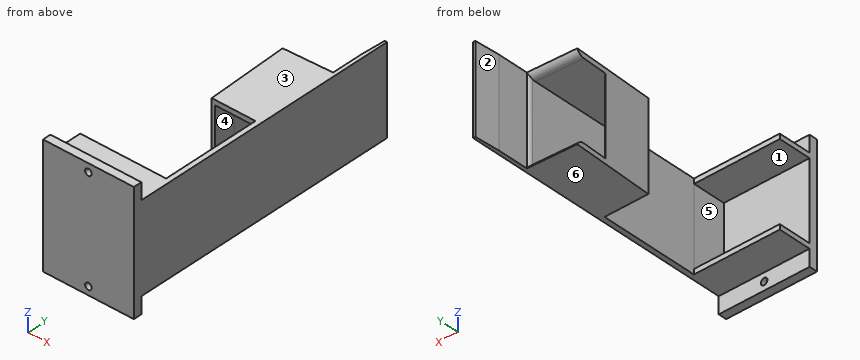
```python
from build123d import *

# Parameters (mm, degrees)
CROQUIS1_W              = 55
CROQUIS1_H              = 53
CROQUIS1_W_2            = 48.773584906
CROQUIS1_H_2            = 47
SALIENTE_EXTRUIR1_DEPTH = 25
SALIENTE_EXTRUIR2_DEPTH = 160
SALIENTE_EXTRUIR3_DEPTH = 50
SALIENTE_EXTRUIR5_DEPTH = 3
CROQUIS4_W              = 100
CROQUIS4_H              = 30
CORTAR_EXTRUIR1_DEPTH   = 63
CHAFL_N1_SIZE           = 2
CHAFL_N1_SIZE2          = 57.272506566
CROQUIS1_2_W            = 55
CROQUIS1_2_H            = 53
CROQUIS1_2_W_2          = 48.773584906
CROQUIS1_2_H_2          = 47
SALIENTE_EXTRUIR6_DEPTH = 5
CROQUIS5_W              = 30
CROQUIS5_H              = 60
CORTAR_EXTRUIR2_DEPTH   = 60
CROQUIS1_4_W            = 55
CROQUIS1_4_H            = 10
CROQUIS1_4_R            = 2
SALIENTE_EXTRUIR7_DEPTH = 5
CROQUIS6_W              = 53
CROQUIS6_H              = 15
CORTAR_EXTRUIR3_DEPTH   = 5
CHAFL_N2_SIZE           = 30
CHAFL_N2_SIZE_2         = 1.572233378
CHAFL_N3_SIZE           = 5
CHAFL_N3_SIZE2          = 0.881634904
CROQUIS7_W              = 47
CROQUIS7_H              = 20
CORTAR_EXTRUIR4_DEPTH   = 40
CROQUIS8_W              = 47
CROQUIS8_H              = 40
CORTAR_EXTRUIR5_DEPTH   = 10
CORTAR_EXTRUIR6_DEPTH   = 70
REDONDEO3_R             = 5
REDONDEO5_R             = 5


with BuildPart() as part:
    # Croquis1 → Saliente-Extruir1 (new body)
    with BuildSketch(Plane(origin=(0, 0, 0), x_dir=(1, 0, 0), z_dir=(0, 1, 0))):
        Rectangle(CROQUIS1_W, CROQUIS1_H)
        Rectangle(CROQUIS1_W_2, CROQUIS1_H_2, mode=Mode.SUBTRACT)
    extrude(amount=SALIENTE_EXTRUIR1_DEPTH)

    # Croquis2 → Saliente-Extruir2 (add)
    with BuildSketch(Plane(origin=(0, 25, 0), x_dir=(1, 0, 0), z_dir=(0, 1, 0))):
        Polygon((0, 23.5), (0, 26.5), (27.5, 26.5), (27.5, -26.5), (0, -26.5), (0, -23.5), (24.386792453, -23.5), (24.386792453, 23.5), align=None)
    extrude(amount=SALIENTE_EXTRUIR2_DEPTH)



with BuildPart() as body_2:
    # Croquis3 → Saliente-Extruir3 (new body)
    with BuildSketch(Plane(origin=(0, 0, 23.5), x_dir=(-1, 0, 0), z_dir=(0, 0, -1))):
        Polygon((0, 155), (5, 155), (2, 85), (0, 85), align=None)
    extrude(amount=SALIENTE_EXTRUIR3_DEPTH)


with BuildPart() as part_1:
    add(part.part)

    add(body_2.part)  # Saliente-Extruir5 merges body 2
    # Croquis3<4> → Saliente-Extruir5 (add)
    with BuildSketch(Plane(origin=(0, 0, 23.5), x_dir=(-1, 0, 0), z_dir=(0, 0, -1))):
        Polygon((0, 155), (5, 155), (2, 85), (0, 85), align=None)
    extrude(amount=-SALIENTE_EXTRUIR5_DEPTH)

    # Croquis4 → Cortar-Extruir1 (cut)
    with BuildSketch(Plane(origin=(0, 0, -26.5), x_dir=(-1, 0, 0), z_dir=(0, 0, -1))):
        with Locations((25.5, 170)):
            Rectangle(CROQUIS4_W, CROQUIS4_H)
    extrude(amount=-CORTAR_EXTRUIR1_DEPTH, mode=Mode.SUBTRACT)

    # Chaflán1
    chafl_n1_edges = [part_1.edges().sort_by_distance(p)[0] for p in [
        (0, 155, 0),
    ]]
    chafl_n1_side = [part_1.faces().sort_by_distance(p)[0] for p in [
        (9.75, 155, -25.893431785),
    ]]
    chamfer(chafl_n1_edges, length=CHAFL_N1_SIZE, length2=CHAFL_N1_SIZE2, reference=chafl_n1_side[0])

    # Croquis1<2> → Saliente-Extruir6 (add)
    # profile 1 of 2: a face of its own
    with BuildSketch(Plane(origin=(0, 0, 0), x_dir=(1, 0, 0), z_dir=(0, 1, 0))):
        Rectangle(CROQUIS1_2_W, CROQUIS1_2_H)
        Rectangle(CROQUIS1_2_W_2, CROQUIS1_2_H_2, mode=Mode.SUBTRACT)
    # profile 2 of 2: a face of its own
    with BuildSketch(Plane(origin=(0, 0, 0), x_dir=(1, 0, 0), z_dir=(0, 1, 0))):
        Rectangle(CROQUIS1_2_W_2, CROQUIS1_2_H_2)
    extrude(amount=SALIENTE_EXTRUIR6_DEPTH)

    # Croquis5 → Cortar-Extruir2 (cut)
    with BuildSketch(Plane(origin=(0, 0, -26.5), x_dir=(-1, 0, 0), z_dir=(0, 0, -1))):
        with Locations((-9.5, 55)):
            Rectangle(CROQUIS5_W, CROQUIS5_H)
    extrude(amount=-CORTAR_EXTRUIR2_DEPTH, mode=Mode.SUBTRACT)

    # Croquis1<4> → Saliente-Extruir7 (add)
    # profile 1 of 2: a face of its own
    with BuildSketch(Plane(origin=(0, 0, 0), x_dir=(1, 0, 0), z_dir=(0, 1, 0))):
        with Locations((0, 31.5)):
            Rectangle(CROQUIS1_4_W, CROQUIS1_4_H)
        with Locations(Location((0, 31.5, 0), (0, 0, 270))):
            Circle(CROQUIS1_4_R, mode=Mode.SUBTRACT)
    # profile 2 of 2: a face of its own
    with BuildSketch(Plane(origin=(0, 0, 0), x_dir=(1, 0, 0), z_dir=(0, 1, 0))):
        with Locations((0, -31.5)):
            Rectangle(CROQUIS1_4_W, CROQUIS1_4_H)
        with Locations(Location((0, -31.5, 0), (0, 0, 270))):
            Circle(CROQUIS1_4_R, mode=Mode.SUBTRACT)
    extrude(amount=SALIENTE_EXTRUIR7_DEPTH)

    # Croquis6 → Cortar-Extruir3 (cut)
    with BuildSketch(Plane.ZY.offset(-24.5)):
        with Locations((0, 177.5)):
            Rectangle(CROQUIS6_W, CROQUIS6_H)
    extrude(amount=-CORTAR_EXTRUIR3_DEPTH, mode=Mode.SUBTRACT)

    # Chaflán2
    # the kernel refuses this chamfer: 30, 1.572233378 mm, written as the material it takes off along each edge
    with BuildSketch(Plane(origin=(24.5, 170, -104.496046635), x_dir=(-0.002013023422382327, -0.9999979738662979, 0), z_dir=(0, 0, 1))) as chafl_n2_piece_1_section:
        Polygon((CHAFL_N2_SIZE * 0.999997973866, CHAFL_N2_SIZE * 0.00201302342238), (-CHAFL_N2_SIZE_2 * 0.00201302342301, CHAFL_N2_SIZE_2 * 0.999997974179), (0, 0), align=None)
    chafl_n2_piece_1 = extrude(amount=208.992093269, mode=Mode.PRIVATE)
    chafl_n2_piece_1 = split(chafl_n2_piece_1, bisect_by=Plane(origin=(25.111424092, 155, 0), z_dir=(0, 1, 0)), keep=Keep.TOP, mode=Mode.PRIVATE)
    add(chafl_n2_piece_1, mode=Mode.SUBTRACT)

    # Chaflán3
    chafl_n3_edges = [part_1.edges().sort_by_distance(p)[0] for p in [
        (24.386792453, 155, 0),
    ]]
    chafl_n3_side = [part_1.faces().sort_by_distance(p)[0] for p in [
        (24.386792453, 120, 0),
    ]]
    chamfer(chafl_n3_edges, length=CHAFL_N3_SIZE, length2=CHAFL_N3_SIZE2, reference=chafl_n3_side[0])

    # Croquis7 → Cortar-Extruir4 (cut)
    with BuildSketch(Plane.ZY.offset(27.5)):
        with Locations((0, 15)):
            Rectangle(CROQUIS7_W, CROQUIS7_H)
    extrude(amount=-CORTAR_EXTRUIR4_DEPTH, mode=Mode.SUBTRACT)

    # Croquis8 → Cortar-Extruir5 (cut)
    with BuildSketch(Plane(origin=(1.639845182, 0.070279079, 0), x_dir=(0, 0, 1), z_dir=(-0.9990828958176697, -0.04281783839218585, 0))):
        with Locations((0, 135.071938044)):
            Rectangle(CROQUIS8_W, CROQUIS8_H)
    extrude(amount=-CORTAR_EXTRUIR5_DEPTH, mode=Mode.SUBTRACT)

    # Croquis9 → Cortar-Extruir6 (cut)
    with BuildSketch(Plane.XY.offset(26.5)):
        Polygon((-5, 155), (25.286116689, 155), (25.286116689, 136.279617509), (-4.143643232, 135.018342084), align=None)
    extrude(amount=-CORTAR_EXTRUIR6_DEPTH, mode=Mode.SUBTRACT)

    # Redondeo3
    # the kernel refuses this fillet: 5 mm, written as the material it takes off along each edge
    with BuildSketch(Plane(origin=(-4.143643232, 135.018342084, 23.5), x_dir=(0, 0, 1), z_dir=(0.9990828958176697, 0.042817838392185704, 0))) as redondeo3_piece_1_section:
        with BuildLine():
            CenterArc((5, 4.582575695), REDONDEO3_R, 180, 66.421821522)
            Line((0, 4.582575695), (-0.1, 4.582575695))
            Line((-0.1, 4.582575695), (-0.1, 0))
            Line((-0.1, 0), (0, -0.1))
            ThreePointArc((0, -0.1), (1.5, -0.1), (2.96, -0.091651514))
            Line((2.96, -0.091651514), (3, 0))
        make_face()
    redondeo3_piece_1 = extrude(amount=40.013064323, mode=Mode.PRIVATE)
    redondeo3_piece_1 = split(redondeo3_piece_1, bisect_by=Plane(origin=(24.386792453, 134.515316135, 24.276456874), z_dir=(-1, 0, 0)), keep=Keep.TOP, mode=Mode.PRIVATE)
    add(redondeo3_piece_1, mode=Mode.SUBTRACT)
    with BuildSketch(Plane(origin=(24.386792453, 136.241075042, 23.5), x_dir=(0.9990828958176863, 0.04281783839180005, 0), z_dir=(0, 0, -1))) as redondeo3_piece_2:
        with BuildLine():
            CenterArc((4.874569404, 3.033807599), REDONDEO3_R, 182.454031675, 34.901674654)
            Line((-0.120845075, 2.819718407), (-0.220753364, 2.815436623))
            Line((-0.220753364, 2.815436623), (-0.09990829, -0.004281784))
            Line((-0.09990829, -0.004281784), (0, -0.1))
            ThreePointArc((0, -0.1), (0.450074884, -0.1), (0.820661375, -0.060676152))
            Line((0.820661375, -0.060676152), (0.900149768, 0))
        make_face()
    extrude(amount=47, mode=Mode.SUBTRACT)
    with BuildSketch(Plane(origin=(35.832724942, 136.731615005, -23.5), x_dir=(0.0428178383921857, -0.9990828958176697, 0), z_dir=(-0.9990828958176697, -0.042817838392185704, 0))) as redondeo3_piece_3_section:
        with BuildLine():
            CenterArc((4.582575695, -5), REDONDEO3_R, 90, 66.421821522)
            Line((0, -3), (-0.091651514, -2.96))
            ThreePointArc((-0.091651514, -2.96), (-0.1, -1.5), (-0.1, 0))
            Line((-0.1, 0), (0, 0.1))
            Line((0, 0.1), (4.582575695, 0.1))
            Line((4.582575695, 0.1), (4.582575695, 0))
        make_face()
    redondeo3_piece_3 = extrude(amount=40.013064323, mode=Mode.PRIVATE)
    redondeo3_piece_3 = split(redondeo3_piece_3, bisect_by=Plane(origin=(24.386792453, 134.515316135, -24.276456874), z_dir=(-1, 0, 0)), keep=Keep.TOP, mode=Mode.PRIVATE)
    add(redondeo3_piece_3, mode=Mode.SUBTRACT)
    with BuildSketch(Plane(origin=(-4.143643232, 135.018342084, 23.5), x_dir=(0, 0, 1), z_dir=(0.9990828958176697, 0.042817838392185704, 0))) as redondeo3_piece_4a_section:
        with BuildLine():
            CenterArc((5, 4.582575695), REDONDEO3_R, 180, 66.421821522)
            Line((0, 4.582575695), (-0.1, 4.582575695))
            Line((-0.1, 4.582575695), (-0.1, 0))
            Line((-0.1, 0), (0, -0.1))
            ThreePointArc((0, -0.1), (1.5, -0.1), (2.96, -0.091651514))
            Line((2.96, -0.091651514), (3, 0))
        make_face()
    redondeo3_piece_4a = extrude(amount=40.013064323, mode=Mode.PRIVATE)
    redondeo3_piece_4a = split(redondeo3_piece_4a, bisect_by=Plane(origin=(24.386792453, 135.366576267, 24.274229372), z_dir=(1, 0, 0)), keep=Keep.TOP, mode=Mode.PRIVATE)
    with BuildSketch(Plane(origin=(24.386792453, 136.241075042, 30.555766892), x_dir=(0.9990828958176863, 0.04281783839180005, 0), z_dir=(0, 0, -1))) as redondeo3_piece_4b_section:
        with BuildLine():
            CenterArc((4.874569404, 3.033807599), REDONDEO3_R, 182.454031675, 34.901674654)
            Line((-0.120845075, 2.819718407), (-0.220753364, 2.815436623))
            Line((-0.220753364, 2.815436623), (-0.09990829, -0.004281784))
            Line((-0.09990829, -0.004281784), (0, -0.1))
            ThreePointArc((0, -0.1), (0.450074884, -0.1), (0.820661375, -0.060676152))
            Line((0.820661375, -0.060676152), (0.900149768, 0))
        make_face()
    redondeo3_piece_4b = extrude(amount=54.055766892, mode=Mode.PRIVATE)
    redondeo3_piece_4b = split(redondeo3_piece_4b, bisect_by=Plane(origin=(24.583130189, 135.440658169, 23.5), z_dir=(0, 0, 1)), keep=Keep.TOP, mode=Mode.PRIVATE)
    redondeo3_piece_4 = redondeo3_piece_4a & redondeo3_piece_4b
    add(redondeo3_piece_4, mode=Mode.SUBTRACT)
    with BuildSketch(Plane(origin=(35.832724942, 136.731615005, -23.5), x_dir=(0.0428178383921857, -0.9990828958176697, 0), z_dir=(-0.9990828958176697, -0.042817838392185704, 0))) as redondeo3_piece_5a_section:
        with BuildLine():
            CenterArc((4.582575695, -5), REDONDEO3_R, 90, 66.421821522)
            Line((0, -3), (-0.091651514, -2.96))
            ThreePointArc((-0.091651514, -2.96), (-0.1, -1.5), (-0.1, 0))
            Line((-0.1, 0), (0, 0.1))
            Line((0, 0.1), (4.582575695, 0.1))
            Line((4.582575695, 0.1), (4.582575695, 0))
        make_face()
    redondeo3_piece_5a = extrude(amount=40.013064323, mode=Mode.PRIVATE)
    redondeo3_piece_5a = split(redondeo3_piece_5a, bisect_by=Plane(origin=(24.386792453, 135.366576267, -24.274229372), z_dir=(1, 0, 0)), keep=Keep.TOP, mode=Mode.PRIVATE)
    with BuildSketch(Plane(origin=(24.386792453, 136.241075042, 23.5), x_dir=(0.9990828958176863, 0.04281783839180005, 0), z_dir=(0, 0, -1))) as redondeo3_piece_5b_section:
        with BuildLine():
            CenterArc((4.874569404, 3.033807599), REDONDEO3_R, 182.454031675, 34.901674654)
            Line((-0.120845075, 2.819718407), (-0.220753364, 2.815436623))
            Line((-0.220753364, 2.815436623), (-0.09990829, -0.004281784))
            Line((-0.09990829, -0.004281784), (0, -0.1))
            ThreePointArc((0, -0.1), (0.450074884, -0.1), (0.820661375, -0.060676152))
            Line((0.820661375, -0.060676152), (0.900149768, 0))
        make_face()
    redondeo3_piece_5b = extrude(amount=54.055766892, mode=Mode.PRIVATE)
    redondeo3_piece_5b = split(redondeo3_piece_5b, bisect_by=Plane(origin=(24.583130189, 135.440658169, -23.5), z_dir=(0, 0, -1)), keep=Keep.TOP, mode=Mode.PRIVATE)
    redondeo3_piece_5 = redondeo3_piece_5a & redondeo3_piece_5b
    add(redondeo3_piece_5, mode=Mode.SUBTRACT)

    # Redondeo5
    # the kernel refuses this fillet: 5 mm, written as the material it takes off along each edge
    with BuildSketch(Plane(origin=(-0.608459404, 115.151491041, -23.5), x_dir=(-0.9990828958176692, -0.04281783839219633, 0), z_dir=(0, 0, 1))) as redondeo5_piece_1:
        with BuildLine():
            CenterArc((5.035114331, 4.411291484), REDONDEO5_R, 179.545968325, 62.370023628)
            Line((0.035271319, 4.450912808), (0, 0))
            Line((0, 0), (2.681286079, 0))
        make_face()
    extrude(amount=47, mode=Mode.SUBTRACT)


solid = part_1.part
```
Work out the finished part from the listing and answer in its coordinate system (mm). Face numbers are marked on the shaded views. A direction names the side the tool comes from. Coordinates: 2 decimals unless noted, no trailing zeros. Loops run counter-clockwise (first coordinate to the right, second up) from the corner with the lowest first, then second, coordinate; pieces in that order, holes last.
1) Section C-C (y = 20) is taken. Give the vertices of the cut face in (x, z), plus the area to 3 significant figures.
Results:
outline: (-27.5, -26.5) - (27.5, -26.5) - (27.5, 26.5) - (-27.5, 26.5) - (-27.5, 23.5) - (24.39, 23.5) - (24.39, -23.5) - (-27.5, -23.5) - close
area: 476 mm2
2) Section A-A (y = 92) is taken. Give the vertices of the cut face in (x, z), plus the area to 3 significant figures.
Results:
outline: (-2.3, -26.5) - (27.5, -26.5) - (27.5, 26.5) - (-2.3, 26.5) - close; hole (0, -23.5) - (24.39, -23.5) - (24.39, 23.5) - (0, 23.5) - close
area: 433 mm2
3) Section D-D (z = 8) is taken. Give the vertices of the cut face in (x, y).
Results:
outline: (-27.5, 0) - (27.5, 0) - (27.5, 170) - (26.07, 170) - (25.29, 155) - (25.29, 136.28) arc R5 ccw to (24.39, 133.42) - (24.39, 85) - (24.5, 85) - (24.5, 25) - (24.39, 25) - (24.39, 5) - (-27.5, 5) - close; (-3.29, 115.04) - (-2, 85) - (0, 85) - (0, 97.73) - (-0.45, 110.7) arc R5 ccw to start
4) Flat-ended cylindrical pins translate along their axes: pin 1 (15.5 mm diameter, centred on x = 2, z = 4, fed in from +Y); pin 2 (10 mm diameter, centred on x = -13, y = 19.5, fed in from +Z); pin 3 (16 mm diameter, centred on y = 60, z = 10, fed in from -X); pin 4 (13 mm diameter, centred on x = 13, z = 10.5, fed in from -Y). Find the tip coordinate at first contact, or state that the pin passes through.
Results:
pin 1: stops at y = 115.04
pin 2: stops at z = 26.5
pin 3: stops at x = 24.5
pin 4: stops at y = 0
5) Section B-B (z = -31.5) is taken. Give the vertices of the cut face in (x, y), plus the area to 3 significant figures.
Results:
outline: (-27.5, 0) - (-2, 0) - (-2, 5) - (-27.5, 5) - close; (2, 0) - (27.5, 0) - (27.5, 5) - (2, 5) - close
area: 255 mm2
6) Consider probe 1 along X at (y, z) = (3.25, -31.5); probe 2 along Z at (x, y) = (5, 98); probe 3 along Y at (x, z) = (-5, 20). Determine where each line is inside the solid, lowest interval first.
Results:
probe 1: x = -27.5 to -2, 2 to 27.5
probe 2: z = -26.5 to -23.5, 23.5 to 26.5
probe 3: y = 0 to 5
7) For a pull along Z with two mould halves and no side action, classify the marked faces 1, 2 and 3 as +Z half, -Z half, draft (parallel to the pull), parting line (faces both ways), or undercut.
Results:
face 1: undercut
face 2: draft
face 3: +Z half
8) For the marked faces 4, 5 and 6, determine the directions among +Z, -Z, +X, -X, +Y, -Y from which every point of the face is accessible in a straight line to the end or side of a thin tool.
Results:
face 4: +Y
face 5: -X, +Y
face 6: -Z, +X, -X, +Y
